Read the model definition and answer for the solid it produces. Units are mm, in the model's axes. A direction names the side the tool comes from. Give positions to 0.01 mm unless a question says otherwise; leave off trailing zeros. Order: outer loops, then holes, each group sorted by start corner. A loop starts at its lowest first (then second) coordinate and runs counter-clockwise, first axis right, second up. Notation, with made-up numbers: M 4.25,70 L 58.25,70 A29 cw 58.25,96 Z; hole C 38.5,17 d10. An arc over 180 degrees is marked long. One line per item, written item: value.
from build123d import *

# Parameters (mm, degrees)
F0_W     = 7.2
F0_H     = 3.5
F0_W_2   = 3.5
F0_H_2   = 7.2
F1_DEPTH = 8


with BuildPart() as f1:
    # F0 (on Top) → F1 (new body)
    with BuildSketch(Plane.XY):
        with BuildLine():
            ThreePointArc((-5, 5), (-3.535534, 1.464466), (0, 0))
            Line((0, 0), (16.1, 0))
            Line((16.1, 0), (16.1, -16.1))
            ThreePointArc((16.1, -16.1), (17.564466, -19.635534), (21.1, -21.1))
            Line((21.1, -21.1), (27.1, -21.1))
            ThreePointArc((27.1, -21.1), (30.635534, -19.635534), (32.1, -16.1))
            Line((32.1, -16.1), (32.1, 0))
            Line((32.1, 0), (59, 0))
            Line((59, 0), (59, 16))
            Line((59, 16), (32.1, 16))
            Line((32.1, 16), (32.1, 32.1))
            ThreePointArc((32.1, 32.1), (30.635534, 35.635534), (27.1, 37.1))
            Line((27.1, 37.1), (21.1, 37.1))
            ThreePointArc((21.1, 37.1), (17.564466, 35.635534), (16.1, 32.1))
            Line((16.1, 32.1), (16.1, 16))
            Line((16.1, 16), (0, 16))
            ThreePointArc((0, 16), (-3.535534, 14.535534), (-5, 11))
            Line((-5, 11), (-5, 5))
        make_face()
        with Locations((24.1, -15.35)):
            Rectangle(F0_W, F0_H, mode=Mode.SUBTRACT)
        with Locations((0.75, 8)):
            Rectangle(F0_W_2, F0_H_2, mode=Mode.SUBTRACT)
        Polygon((30.1, -3.6), (30.1, -11.6), (18.1, -11.6), (18.1, -3.6), (24.1, 3.8), align=None, mode=Mode.SUBTRACT)
        Polygon((12.5, 2), (4.5, 2), (4.5, 14), (12.5, 14), (19.9, 8), align=None, mode=Mode.SUBTRACT)
        Polygon((18.1, 19.6), (18.1, 27.6), (30.1, 27.6), (30.1, 19.6), (24.1, 12.2), align=None, mode=Mode.SUBTRACT)
        with Locations((24.1, 31.35)):
            Rectangle(F0_W, F0_H, mode=Mode.SUBTRACT)
    extrude(amount=F1_DEPTH)


solid = f1.part
1) Consider probe 1 along X at (y, z) = (23.5, 5); probe 2 along Y at (x, z) = (12, 5.5); probe 3 along Y at (x, z) = (25.5, 7.5). Determine where each line is inside the solid, lowest interval first.
Reported:
probe 1: x = 16.1 to 18.1, 30.1 to 32.1
probe 2: y = 0 to 2, 14 to 16
probe 3: y = -21.1 to -17.1, -13.6 to -11.6, 2.07 to 13.93, 27.6 to 29.6, 33.1 to 37.1
2) Find section D-D, the plane x = 53. Write down the section's boundary in (y, z).
Reported:
outline: M 0,0 L 16,0 L 16,8 L 0,8 Z
3) Find section A-A, the plane y = 31. Write down the section's boundary in (x, z), plus the area to 3 significant figures.
Reported:
outline: M 16.1,0 L 20.5,0 L 20.5,8 L 16.1,8 Z; M 27.7,0 L 32.1,0 L 32.1,8 L 27.7,8 Z
area: 70.4 mm^2
4) Determine the mould class of faces 6 (the face through (16.1, 24, 4)), 7 (the face through (1, 4.4, 4)), 8 (the face through (24, 37.1, 4)) for opening direction Y: +Y half, -Y half, draft (parallel to the pull), parting line (faces both ways), or undercut.
Reported:
face 6: draft
face 7: undercut
face 8: +Y half
5) Each of these flat-tipped pins is pushed along its axis until it touches: pin 1 Ø1.8 at (y, z) = (31.5, 4) entering from +X; pin 2 Ø2.5 at (y, z) = (-6.5, 2.5) entering from -X; pin 3 Ø4 at (x, z) = (10.5, 5) entering from +Y. Where does it stop, or does it pass through?
Reported:
pin 1: stops at x = 32.1
pin 2: stops at x = 16.1
pin 3: stops at y = 16
6) Find section B-B, the plane x = 11. Write down the section's boundary in (y, z), plus the area to 3 significant figures.
Reported:
outline: M 0,0 L 2,0 L 2,8 L 0,8 Z; M 14,0 L 16,0 L 16,8 L 14,8 Z
area: 32.0 mm^2
7) Find section C-C, the plane z = 4.5. Count the separate pieces of the cut face and the enclosed holes in it, plus the area to 3 significant figures.
Reported:
separate pieces: 1
enclosed holes: 6
area: 1,170 mm^2
8) Which of the six approach directions +Z, -Z, +X, -X, +Y, -Y give full straight-line access (tool end or side, diameter ignored) to faces 1 (the face through (59, 8, 4)), 2 (the face through (32.1, -8, 4)), 3 (the face through (16.1, -8, 4)), 4 (the face through (24, -17.1, 4)), 5 (the face through (32.1, 24, 4))?
Reported:
face 1: +Z, -Z, +X, +Y, -Y
face 2: +Z, -Z, +X, -Y
face 3: +Z, -Z, -X, -Y
face 4: +Z, -Z
face 5: +Z, -Z, +X, +Y
